```python
from build123d import *

# Parameters (mm, degrees)
PAD002_DEPTH               = 2
PAD002_MIRRORED004_2_DEPTH = 2
POLARPATTERN004_COUNT      = 3


with BuildPart() as part:
    # Sketch012 → Pad002 (new body)
    with BuildSketch(Plane.XY):
        with BuildLine():
            Line((0, 0), (36.418579, 21.026276))
            ThreePointArc((14.4, 90), (21.694701, 54.327325), (36.418579, 21.026276))
            Line((14.4, 90), (0, 90))
            Line((0, 90), (0, 0))
        make_face()
    pad002 = extrude(amount=PAD002_DEPTH)

    # Sketch012 Mirrored004 2 → Pad002 Mirrored004 2 (add)
    with BuildSketch(Plane(origin=(0, 0, 0), x_dir=(-1, 0, 0), z_dir=(0, 0, -1))):
        with BuildLine():
            Line((0, 0), (36.418579, 21.026276))
            ThreePointArc((14.4, 90), (21.694701, 54.327325), (36.418579, 21.026276))
            Line((14.4, 90), (0, 90))
            Line((0, 90), (0, 0))
        make_face()
    pad002_mirrored004_2 = extrude(amount=-PAD002_MIRRORED004_2_DEPTH)

    # PolarPattern004: Pad002, Pad002 Mirrored004 2 ×3 about axis
    polarpattern004_axis = Axis((0, 0, 0), (0, 0, 1))
    for i in range(1, POLARPATTERN004_COUNT):
        add(pad002.rotate(polarpattern004_axis, i * 360 / POLARPATTERN004_COUNT))
        add(pad002_mirrored004_2.rotate(polarpattern004_axis, i * 360 / POLARPATTERN004_COUNT))


solid = part.part
```
Build history of the part. All positions in model axes, mm. Round coordinates to 2 decimals unless told otherwise and drop trailing zeros. Write each loop counter-clockwise with the first axis right and the second up, starting at its lowest first coordinate (ties: lowest second). Pieces come first, ordered by that corner, then holes.
1) Band-saw the part on B-B, the plane x = -22. List the corners of the cut face in (y, z), and give its area (3 significant figures).
2) Band-saw the part on A-A, the plane z = 0.6. List the corners of the cut face in (x, y), and give its area (3 significant figures).
3) Drill centre lines: probe 1 along Y at (x, z) = (3, 0.45); probe 2 along X at (y, z) = (2.5, 0.8); probe 3 along X at (y, z) = (76, 0.9). Where is each one in solid material? Low to high.
4) Band-saw the part on C-C, the plane y = -11. List the corners of the cut face in (x, z).
Ans:
1. outline: (-43.48, 0) - (53.38, 0) - (53.38, 2) - (-43.48, 2) - close
1. area: 194 mm2
2. outline: (-85.14, -32.53) - (-70.74, -57.47) arc R170 cw to (0, -42.05) arc R170 cw to (70.74, -57.47) - (85.14, -32.53) arc R170 cw to (36.42, 21.03) arc R170 cw to (14.4, 90) - (-14.4, 90) arc R170 cw to (-36.42, 21.03) arc R170 cw to start
2. area: 11,700 mm2
3. probe 1: y = -42.08 to 90
3. probe 2: x = -48.8 to 48.8
3. probe 3: x = -16.32 to 16.32
4. outline: (-60.33, 0) - (60.33, 0) - (60.33, 2) - (-60.33, 2) - close
